from build123d import *

# Parameters (mm, degrees)
MODEL_R             = 1.2
MODEL_W             = 11
MODEL_H             = 5.35
MODEL_W_2           = 5.35
MODEL_H_2           = 9
BOSS_EXTRUDE1_DEPTH = 5.35


with BuildPart() as part:
    # Model → Boss-Extrude1 (new body)
    with BuildSketch(Plane.XY):
        with BuildLine():
            Line((0, 0), (45.001, 0))
            Line((45.001, 0), (45.001, -5.35))
            Line((45.001, -5.35), (74.667, -5.35))
            Line((74.667, -5.35), (74.667, 0))
            Line((74.667, 0), (119.667, 0))
            Line((119.667, 0), (119.667, -5.35))
            Line((119.667, -5.35), (149.333, -5.35))
            Line((149.333, -5.35), (149.333, 0))
            Line((149.333, 0), (194.333, 0))
            Line((194.333, 0), (194.333, -5.35))
            Line((194.333, -5.35), (223.999, -5.35))
            Line((223.999, -5.35), (223.999, 0))
            Line((223.999, 0), (269, 0))
            Line((269, 0), (269, 25.85))
            ThreePointArc((269, 25.85), (266.071067812, 32.921067812), (259, 35.85))
            Line((259, 35.85), (150, 35.85))
            ThreePointArc((150, 35.85), (142.928932188, 38.778932188), (140, 45.85))
            Line((140, 45.85), (140, 48.85))
            ThreePointArc((140, 48.85), (137.071067812, 55.921067812), (130, 58.85))
            Line((130, 58.85), (10, 58.85))
            ThreePointArc((10, 58.85), (2.928932188, 55.921067812), (0, 48.85))
            Line((0, 48.85), (0, 0))
        make_face()
        with Locations((37.23, 42.15)):
            Circle(MODEL_R, mode=Mode.SUBTRACT)
        with Locations((88.03, 56.35)):
            Circle(MODEL_R, mode=Mode.SUBTRACT)
        with Locations((89.33, 8.35)):
            Circle(MODEL_R, mode=Mode.SUBTRACT)
        with Locations((37.23, 14.25)):
            Circle(MODEL_R, mode=Mode.SUBTRACT)
        with Locations((13, 29.675)):
            Rectangle(MODEL_W, MODEL_H, mode=Mode.SUBTRACT)
        with Locations((52, 29.675)):
            Rectangle(MODEL_W, MODEL_H, mode=Mode.SUBTRACT)
        with Locations((121, 29.675)):
            Rectangle(MODEL_W, MODEL_H, mode=Mode.SUBTRACT)
        with Locations((160, 29.675)):
            Rectangle(MODEL_W, MODEL_H, mode=Mode.SUBTRACT)
        with Locations((41.675, 13.5)):
            Rectangle(MODEL_W_2, MODEL_H_2, mode=Mode.SUBTRACT)
        with Locations((131.325, 13.5)):
            Rectangle(MODEL_W_2, MODEL_H_2, mode=Mode.SUBTRACT)
        with BuildLine():
            Line((124.21, 54.85), (132.21, 54.85))
            ThreePointArc((132.21, 54.85), (132.563553391, 54.703553391), (132.71, 54.35))
            Line((132.71, 54.35), (132.71, 45.35))
            ThreePointArc((132.71, 45.35), (132.563553391, 44.996446609), (132.21, 44.85))
            Line((132.21, 44.85), (124.21, 44.85))
            ThreePointArc((124.21, 44.85), (123.856446609, 44.996446609), (123.71, 45.35))
            Line((123.71, 45.35), (123.71, 54.35))
            ThreePointArc((123.71, 54.35), (123.856446609, 54.703553391), (124.21, 54.85))
        make_face(mode=Mode.SUBTRACT)
    extrude(amount=BOSS_EXTRUDE1_DEPTH)


solid = part.part
Part model, mm, in its own coordinate system. A direction names the side the tool comes from. Round coordinates to 2 decimals unless told otherwise and drop trailing zeros. Write each loop counter-clockwise with the first axis right and the second up, starting at its lowest first coordinate (ties: lowest second). Pieces come first, ordered by that corner, then holes. Notation, with made-up numbers: M 47.5,56.5 L 80.5,56.5 A20 cw 80.5,85.5 Z; hole C 71,82 d1. An arc over 180 degrees is marked long. Return JSON: item names as keys, results as strings. Group by question number.
(1) Saw through at A-A on x = 207.5. Write the cut outline in (y, z).
(2) Saw through at B-B on z = 1. Count the separate pieces of the cut face and the enclosed holes in it, then the cut area to 3 significant figures.
(3) Pin check, flat tips, straight feed: pin 1 Ø2.5 at (x, z) = (222, 4) entering from +Y; pin 2 Ø2.5 at (y, z) = (-2, 4) entering from +X; pin 3 Ø2.5 at (x, z) = (20.5, 3) entering from -Y. Stop position of each tip, or through.
(4) Which spindle directions (+Z, -Z, +X, -X, +Y, -Y) get a long thin tool onto all of the face, cutting with end or side? Do faces 5 (the face through (119.667, -3, 3)), 6 (the face through (134, -5.35, 3)), 7 (the face through (126.5, 30, 3)). Say none if no direction does.
(5) Drill centre lines: probe 1 along X at (y, z) = (17.5, 4.6); probe 2 along Y at (x, z) = (37.23, 2.35); probe 3 along Y at (x, z) = (88.03, 1.7). Where is each one in solid material? Low to high.
(6) Two-plate mould, pull along X, no slides. Class faces 1 (the face through (42, 18, 3)), 2 (the face through (266.15, 32.84, 2.64)), 3 (the face through (3.01, 56, 2.64)), 4 (the face through (71, 58.85, 3)): +X half, -X half, draft (parallel to the pull), parting line (faces both ways), or undercut.
Returned:
{
 "1": {"outline": "M -5.35,0 L 35.85,0 L 35.85,5.35 L -5.35,5.35 Z"},
 "2": {"separate pieces": "1", "enclosed holes": "11", "area": "12,900 mm²"},
 "3": {"pin 1": "y = 35.85", "pin 2": "x = 224", "pin 3": "y = 0"},
 "4": {"face 5": "+Z, -Z, -Y", "face 6": "+Z, -Z, +X, -X, -Y", "face 7": "+Z, -Z"},
 "5": {"probe 1": "0 to 39, 44.35 to 128.65, 134 to 269", "probe 2": "0 to 13.05, 15.45 to 40.95, 43.35 to 58.85", "probe 3": "0 to 55.15, 57.55 to 58.85"},
 "6": {"face 1": "undercut", "face 2": "+X half", "face 3": "-X half", "face 4": "draft"}
}
